Here's how the part is built. I have some questions about the finished solid (model axes, mm). Round coordinates to 2 decimals unless told otherwise and drop trailing zeros. Write each loop counter-clockwise with the first axis right and the second up, starting at its lowest first coordinate (ties: lowest second). Pieces come first, ordered by that corner, then holes. Notation, with made-up numbers: (49, 53.25) - (75, 53.25) arc R21 cw to (75, 90.25) - close; hole circle Ø10 at (25.5, 52). An arc over 180 degrees is marked (long way). Write item = value, one per line. Start each with the question number.
Item 1: For P1, Ø6, axis at x = -40.5, y = 37.5, coming from the +Z side; P2, Ø1, axis at y = 37, z = 2, coming from the -X side; P3, Ø0.7, axis at y = -52, z = 1.5, coming from the +X side; P4, Ø1.2, axis at y = 51.5, z = 1.5, coming from the -X side, each with a flat end and sliding along its axis, tell me the tip position at first contact or that it passes through.
Item 2: If I drill on line 1 along Y through (x, z) = (0, 1.9); line 2 along X through (y, z) = (25.5, 0.55); line 3 along X through (y, z) = (-29.5, 2.75), over which ranges is the centre line in solid material (lowest first)? Write a range as [from, to].
Item 3: If we section it at B-B (y = 0): Please give me the cut outline in (x, z), and give its area (3 significant figures).
Item 4: If we section it at A-A (x = 0): Please give me the cut outline in (y, z).
```python
from build123d import *

# Parameters (mm, degrees)
BOSS_EXTRUDE1_DEPTH = 3
SKETCH1_R           = 40
CUT_EXTRUDE1_DEPTH  = 76.086906122


with BuildPart() as part:
    # Base_Sketch → Boss-Extrude1 (new body)
    with BuildSketch(Plane.XY):
        with BuildLine():
            Line((-8.603981625, 52.439957176), (-8.603981625, 50.01533765))
            ThreePointArc((-8.603981625, 50.01533765), (-15.682612465, 48.266118202), (-22.437510505, 45.520551648))
            Line((-22.437510505, 45.520551648), (-23.862666105, 47.48211005))
            Line((-23.862666105, 47.48211005), (-24.825537526, 47.634613901))
            Line((-24.825537526, 47.634613901), (-37.631696962, 38.33039445))
            Line((-37.631696962, 38.33039445), (-37.784200813, 37.36752303))
            Line((-37.784200813, 37.36752303), (-36.359045213, 35.405964628))
            ThreePointArc((-36.359045213, 35.405964628), (-41.057612465, 29.830101554), (-44.908636245, 23.638462104))
            Line((-44.908636245, 23.638462104), (-47.214586445, 24.387710742))
            Line((-47.214586445, 24.387710742), (-48.083205302, 23.945127328))
            Line((-48.083205302, 23.945127328), (-52.974722942, 8.890584019))
            Line((-52.974722942, 8.890584019), (-52.532139528, 8.021965161))
            Line((-52.532139528, 8.021965161), (-50.226189328, 7.272716523))
            ThreePointArc((-50.226189328, 7.272716523), (-50.75, 0), (-50.226189328, -7.272716523))
            Line((-50.226189328, -7.272716523), (-52.532139528, -8.021965161))
            Line((-52.532139528, -8.021965161), (-52.974722942, -8.890584019))
            Line((-52.974722942, -8.890584019), (-48.083205302, -23.945127328))
            Line((-48.083205302, -23.945127328), (-47.214586445, -24.387710742))
            Line((-47.214586445, -24.387710742), (-44.908636245, -23.638462104))
            ThreePointArc((-44.908636245, -23.638462104), (-41.057612465, -29.830101554), (-36.359045213, -35.405964628))
            Line((-36.359045213, -35.405964628), (-37.784200813, -37.36752303))
            Line((-37.784200813, -37.36752303), (-37.631696962, -38.33039445))
            Line((-37.631696962, -38.33039445), (-24.825537526, -47.634613901))
            Line((-24.825537526, -47.634613901), (-23.862666105, -47.48211005))
            Line((-23.862666105, -47.48211005), (-22.437510505, -45.520551648))
            ThreePointArc((-22.437510505, -45.520551648), (-15.682612465, -48.266118202), (-8.603981625, -50.01533765))
            Line((-8.603981625, -50.01533765), (-8.603981625, -52.439957176))
            Line((-8.603981625, -52.439957176), (-7.914641797, -53.129297004))
            Line((-7.914641797, -53.129297004), (7.914641797, -53.129297004))
            Line((7.914641797, -53.129297004), (8.603981625, -52.439957176))
            Line((8.603981625, -52.439957176), (8.603981625, -50.01533765))
            ThreePointArc((8.603981625, -50.01533765), (15.682612465, -48.266118202), (22.437510505, -45.520551648))
            Line((22.437510505, -45.520551648), (23.862666105, -47.48211005))
            Line((23.862666105, -47.48211005), (24.825537526, -47.634613901))
            Line((24.825537526, -47.634613901), (37.631696962, -38.33039445))
            Line((37.631696962, -38.33039445), (37.784200813, -37.36752303))
            Line((37.784200813, -37.36752303), (36.359045213, -35.405964628))
            ThreePointArc((36.359045213, -35.405964628), (41.057612465, -29.830101554), (44.908636245, -23.638462104))
            Line((44.908636245, -23.638462104), (47.214586445, -24.387710742))
            Line((47.214586445, -24.387710742), (48.083205302, -23.945127328))
            Line((48.083205302, -23.945127328), (52.974722942, -8.890584019))
            Line((52.974722942, -8.890584019), (52.532139528, -8.021965161))
            Line((52.532139528, -8.021965161), (50.226189328, -7.272716523))
            ThreePointArc((50.226189328, -7.272716523), (50.75, 0), (50.226189328, 7.272716523))
            Line((50.226189328, 7.272716523), (52.532139528, 8.021965161))
            Line((52.532139528, 8.021965161), (52.974722942, 8.890584019))
            Line((52.974722942, 8.890584019), (48.083205302, 23.945127328))
            Line((48.083205302, 23.945127328), (47.214586445, 24.387710742))
            Line((47.214586445, 24.387710742), (44.908636245, 23.638462104))
            ThreePointArc((44.908636245, 23.638462104), (41.057612465, 29.830101554), (36.359045213, 35.405964628))
            Line((36.359045213, 35.405964628), (37.784200813, 37.36752303))
            Line((37.784200813, 37.36752303), (37.631696962, 38.33039445))
            Line((37.631696962, 38.33039445), (24.825537526, 47.634613901))
            Line((24.825537526, 47.634613901), (23.862666105, 47.48211005))
            Line((23.862666105, 47.48211005), (22.437510505, 45.520551648))
            ThreePointArc((22.437510505, 45.520551648), (15.682612465, 48.266118202), (8.603981625, 50.01533765))
            Line((8.603981625, 50.01533765), (8.603981625, 52.439957176))
            Line((8.603981625, 52.439957176), (7.914641797, 53.129297004))
            Line((7.914641797, 53.129297004), (-7.914641797, 53.129297004))
            Line((-7.914641797, 53.129297004), (-8.603981625, 52.439957176))
        make_face()
    extrude(amount=BOSS_EXTRUDE1_DEPTH)

    # Sketch1 → Cut-Extrude1 (cut, through all)
    with BuildSketch(Plane(origin=(0, 0, 0), x_dir=(-1, 0, 0), z_dir=(0, 0, -1))):
        Circle(SKETCH1_R)
    extrude(amount=-CUT_EXTRUDE1_DEPTH, mode=Mode.SUBTRACT)


solid = part.part
```
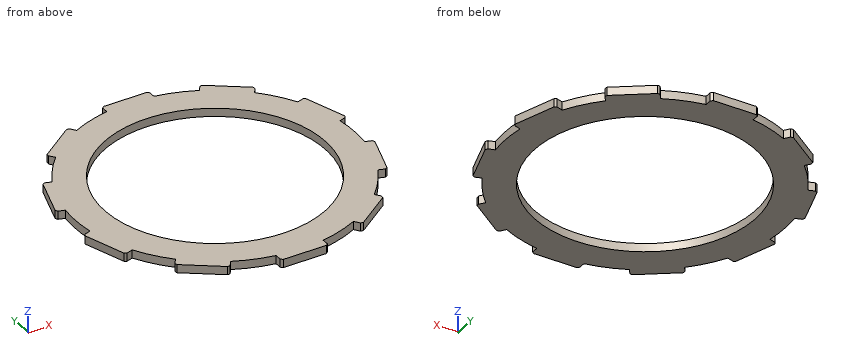
Reply:
q1.P1 = 3
q1.P2 = -37.78
q1.P3 = 8.6
q1.P4 = -8.6
q2.line_1 = [-53.13, -40], [40, 53.13]
q2.line_2 = [-43.88, -30.82], [30.82, 43.88]
q2.line_3 = [-41.3, -27.01], [27.01, 41.3]
q3.outline = (-50.75, 0) - (-40, 0) - (-40, 3) - (-50.75, 3) - close; (40, 0) - (50.75, 0) - (50.75, 3) - (40, 3) - close
q3.area = 64.5 mm2
q4.outline = (-53.13, 0) - (-40, 0) - (-40, 3) - (-53.13, 3) - close; (40, 0) - (53.13, 0) - (53.13, 3) - (40, 3) - close
